Check sheet for the modelled part. Datum: model origin and axes. Units: mm. A direction names the side the tool comes from. Coordinates: 2 decimals unless noted, no trailing zeros. Order: outer loops, then holes, each group sorted by start corner. A loop starts at its lowest first (then second) coordinate and runs counter-clockwise, first axis right, second up.
Autodesk Inventor part; units mm, degrees
ref_plane "Pracovní rovina1" through (0, -5, 0) normal (1, 0, 0) x (0, 0, -1)
ref_plane "YZ Plane" through (0, 0, 0) normal (1, 0, 0) x (0, 1, 0)
ref_plane "XZ Plane" through (0, 0, 0) normal (0, 1, 0) x (-1, 0, 0)
sketch "Náčrt1" plane through (0, 0, 0) normal (0, 0, 1) x (1, 0, 0)
  line L0 (-3.3166, 5) -> (3.3166, 5)
  line L1 (3.3166, -5) -> (-3.3166, -5)
  arc A0 (-3.3166, 5) -> (-6, 0) centre (0, 0) ccw
  arc A1 (6, 0) -> (3.3166, 5) centre (0, 0) ccw
  line L2 (-3.3166, 5) -> (3.3166, -5)
  line L3 (3.3166, 5) -> (-3.3166, -5)
  line L4 (-16, 7) -> (16, 7)
  line L5 (16, 7) -> (16, -5)
  line L6 (16, -5) -> (-16, -5)
  line L7 (-16, -5) -> (-16, 7)
  line L8 (0, 5) -> (0, -5)
  line L9 (-16, 4) -> (-6.9282, 4)
  arc A2 (8, 0) -> (3.873, 7) centre (0, 0) ccw
  line L10 (3.873, 7) -> (-3.873, 7)
  line L11 (-8, 0) -> (-8, -5)
  line L12 (-6, 0) -> (-6, -5)
  line L13 (6, 0) -> (6, -5)
  line L14 (8, 0) -> (8, -5)
  arc A3 (-3.873, 7) -> (-8, 0) centre (0, 0) ccw
  line L15 (6.9282, 4) -> (16, 4)
  point P0 (3.873, 7)
  dimension "d13" = 10
  dimension "d14" = 12
  dimension "d15" = 6
  dimension "d16" = 32
  dimension "d17" = 12
  dimension "d20" = 9
extrude "Vysunutí1" add sketch "Náčrt1" along normal blind 10 contours A0 L12 L6 L11 A3 L4 A2 L14 L13 A1 L0 | L6 L7 L9 A3 L11 | L14 A2 L15 L5 L6
sketch "Náčrt2" plane through (-16, 4, 0) normal (0, 1, 0) x (1, 0, 0)
  line L0 (0, 0) -> (0, -10)
  line L1 (9.0718, -10) -> (0, -10)
  point P0 (16, 0)
  point P1 (4.5, -5)
  dimension "d24" = 4.5
  dimension "d25" = 5
hole "Díra1" at (-11.5, 4, 5) direction (0, -1, 0) diameter 3.5 end through all counterbore diameter 6 counterbore depth 3
ref_plane "Pracovní rovina1" through (0, -5, 0) normal (1, 0, 0) x (0, 0, -1)
mirror "Zrcadlit1" about plane through (0, -5, 0) normal (1, 0, 0) of "Díra1"
move faces "Posunout1" translate (0, 0.5, 0) faces at (-7.2543, -5, 5.0703) (7.2543, -5, 5.0703)
chamfer "Zkosení1" distance 0.5 angle 45 2 edges at (-11.5, 4, 2) (11.5, 4, 2)
properties part number "Držak motoru"
(1) Cross-section at C-C (z = 9.25). Enter the section's corners in (x, y).
Filled in:
outline: (-16, -4.5) - (-6, -4.5) - (-6, 0) arc R6 cw to (-3.32, 5) - (3.32, 5) arc R6 cw to (6, 0) - (6, -4.5) - (16, -4.5) - (16, 4) - (6.93, 4) arc R8 ccw to (3.87, 7) - (-3.87, 7) arc R8 ccw to (-6.93, 4) - (-16, 4) - close
(2) Tool access check on faces 1 (the flat face through (8, 4, 3)), 2 (the flat face through (-16, 0, 5)), 3 (the cylindrical face through (-5.306, 2.801, 4.93)), 4 (the flat face through (10, -4.5, 3.8)), 5 (the cylindrical face through (13.3, 2.2, 2.6)). Record the directions out of +Z, -Z, +X, -X, +Y, -Y that give a thin tool (end or side, any length) a straight path to the whole face; none if there is none.
Filled in:
face 1: +Z, -Z, +X, +Y
face 2: +Z, -Z, -X, +Y, -Y
face 3: +Z, -Z, -Y
face 4: +Z, -Z, +X, -X, -Y
face 5: +Y
(3) Thickness scan on probe 1 along X at (y, z) = (-2.7, 5); probe 2 along Z at (x, y) = (-11.5, 1.65); probe 3 along X at (y, z) = (0, 7.75). Record the ranges inside material, lowest first.
Filled in:
probe 1: x = -16 to -13.25, -9.75 to -6, 6 to 9.75, 13.25 to 16
probe 2: z = 0 to 2, 8 to 10
probe 3: x = -16 to -6, 6 to 16
(4) Cross-section at A-A (x = -11.5). Enter the section's corners in (y, z).
Filled in:
outline: (-4.5, 0) - (4, 0) - (4, 1.5) - (3.5, 2) - (1, 2) - (1, 3.25) - (-4.5, 3.25) - close; (-4.5, 6.75) - (1, 6.75) - (1, 8) - (3.5, 8) - (4, 8.5) - (4, 10) - (-4.5, 10) - close
(5) Cross-section at B-B (z = 5). Count the separate pieces of the cut face and the enclosed holes in it, and give its area (3 significant figures).
Filled in:
separate pieces: 3
enclosed holes: 0
area: 125 mm2
(6) Go/stop test with flat-tipped pins: P1, Ø5, axis at x = 11.5, z = 5, coming from the +Y side; P2, Ø1, axis at x = -6.5, z = 7, coming from the +Y side; P3, Ø2.5, axis at x = 13, z = 3.5, coming from the +Y side. Record where each tip stops, or that it passes through.
Filled in:
P1: stops at y = 1
P2: stops at y = 5.29
P3: stops at y = 3.87
(7) Cross-section at D-D (x = -3). Enter the section's corners in (y, z).
Filled in:
outline: (5, 0) - (7, 0) - (7, 10) - (5, 10) - close
(8) Release check for a two-part mould opening along Z. For faces 6 (the flat face through (9.5, 1, 5)), 7 (the flat face through (-0.2, 5.2, 10)), 8 (the flat face through (-15, 4, 3)) record: +Z half, -Z half, draft (parallel to the pull), parting line (faces both ways), or undercut.
Filled in:
face 6: undercut
face 7: +Z half
face 8: draft
